Input: part model. Units: mm. Frame: model coordinates. A direction names the side the tool comes from. Coordinates: 2 decimals unless noted, no trailing zeros. Order: outer loops, then holes, each group sorted by start corner. A loop starts at its lowest first (then second) coordinate and runs counter-clockwise, first axis right, second up. Notation, with made-up numbers: (11, 48) -> (33, 48) arc R33 ccw to (33, 79) -> close; hole circle Ø1 at (28.25, 21). An arc over 180 degrees is marked (long way). Use one line per item in the form item = value. Start each with the question number.
1) Draft query along X for faces 1 (the flat face through (-133, 2, -17.245)), 2 (the flat face through (-2, 2, 4.205)), 3 (the flat face through (-46.62, 1.57, 10.22)). Return one class per face: pulls with the +X half, pulls with the -X half, needs draft (parallel to the pull), parting line crosses it, or undercut.
2) Access query for faces 4 (the flat face through (-122.093, 2, -2)), 5 (the flat face through (-79, 0, -2)). Directions: +Z, -Z, +X, -X, +Y, -Y. A direction counts if a zero-diameter tool reaches every point of the face in a straight line with its end or side. Return the directions, or none.
3) Section query B-B on z = -7. Output: boundary loops of the cut face in (x, y) (3 decimals).
4) Section query D-D on x = -36.5. Output: boundary loops of the cut face in (y, z) (3 decimals).
5) Section query A-A on x = -141. Output: boundary loops of the cut face in (y, z) (3 decimals).
6) Pin query (flat end, axial travel): pin 1 (7 mm diameter, centred on x = -168.39, z = -7.24, fed in from -Y); pin 2 (1 mm diameter, centred on y = 1.5, z = -4.5, fed in from +X); pin 3 (1.6 mm diameter, centred on y = 1, z = 2, fed in from -X); pin 4 (1 mm diameter, centred on x = -7, y = 2.5, fed in from -Z). Return the tip coordinate at first contact, or that it passes through.
7) Ray query, line 1 along Z through (x, y) = (-125.5, 2.35); line 2 along Z through (x, y) = (-117, 0.7); line 3 along X through (y, z) = (3.05, -9). Return the intervals inside material, ascending.
8) Section query C-C on y = 1.1. Count the separate pieces of the cut face and the enclosed holes in it, then the cut area to 3 significant figures.
from build123d import *

# Parameters (mm, degrees)
SKETCH1_R           = 2.25
SKETCH1_R_2         = 1
SKETCH1_W           = 40.6
SKETCH1_H           = 20.8
SKETCH1_W_2         = 23
SKETCH1_H_2         = 12.9
BOSS_EXTRUDE1_DEPTH = 3.175


with BuildPart() as part:
    # Sketch1 → Boss-Extrude1 (new body)
    with BuildSketch(Plane(origin=(0, 0, 0), x_dir=(1, 0, 0), z_dir=(0, 1, 0))):
        with BuildLine():
            Line((-162.38735588, 17.244652891), (-102.38735588, 17.244652891))
            Line((-102.38735588, 17.244652891), (7.61264412, 12.244652891))
            ThreePointArc((7.61264412, 12.244652891), (17.61264412, 2.244652891), (7.61264412, -7.755347109))
            Line((7.61264412, -7.755347109), (-102.38735588, -12.755347109))
            Line((-102.38735588, -12.755347109), (-162.38735588, -12.755347109))
            ThreePointArc((-162.38735588, -12.755347109), (-177.38735588, 2.244652891), (-162.38735588, 17.244652891))
        make_face()
        with Locations(Location((-168.38735588, 7.244652891, 0), (0, 0, 270))):
            Circle(SKETCH1_R, mode=Mode.SUBTRACT)
        with Locations(Location((-168.38735588, -2.755347109, 0), (0, 0, 270))):
            Circle(SKETCH1_R, mode=Mode.SUBTRACT)
        with Locations(Location((-118.78735588, 7.244652891, 0), (0, 0, 270))):
            Circle(SKETCH1_R, mode=Mode.SUBTRACT)
        with Locations(Location((-118.78735588, -2.755347109, 0), (0, 0, 270))):
            Circle(SKETCH1_R, mode=Mode.SUBTRACT)
        with Locations(Location((-15.58735588, 2.244652891, 0), (0, 0, 270))):
            Circle(SKETCH1_R_2, mode=Mode.SUBTRACT)
        with Locations(Location((11.81264412, 2.244652891, 0), (0, 0, 270))):
            Circle(SKETCH1_R_2, mode=Mode.SUBTRACT)
        with Locations(Location((-42.38735588, 2.244652891, 0), (0, 0, 270))):
            Circle(SKETCH1_R, mode=Mode.SUBTRACT)
        with Locations((-142.392621679, 2.244652891)):
            Rectangle(SKETCH1_W, SKETCH1_H, mode=Mode.SUBTRACT)
        with Locations((-1.88735588, 2.244652891)):
            Rectangle(SKETCH1_W_2, SKETCH1_H_2, mode=Mode.SUBTRACT)
    extrude(amount=BOSS_EXTRUDE1_DEPTH)


solid = part.part
Answers below:
q1.face_1 = needs draft
q1.face_2 = undercut
q1.face_3 = pulls with the +X half
q2.face_4 = +Y, -Y
q2.face_5 = +Z, -Z, +X, -X, -Y
q3.outline = (-176.614, 0) -> (-170.624, 0) -> (-170.624, 3.175) -> (-176.614, 3.175) -> close; (-166.151, 0) -> (-162.693, 0) -> (-162.693, 3.175) -> (-166.151, 3.175) -> close; (-122.093, 0) -> (-121.024, 0) -> (-121.024, 3.175) -> (-122.093, 3.175) -> close; (-116.551, 0) -> (-13.387, 0) -> (-13.387, 3.175) -> (-116.551, 3.175) -> close; (9.613, 0) -> (16.41, 0) -> (16.41, 3.175) -> (9.613, 3.175) -> close
q4.outline = (0, -14.25) -> (3.175, -14.25) -> (3.175, 9.76) -> (0, 9.76) -> close
q5.outline = (0, -17.245) -> (3.175, -17.245) -> (3.175, -12.645) -> (0, -12.645) -> close; (0, 8.155) -> (3.175, 8.155) -> (3.175, 12.755) -> (0, 12.755) -> close
q6.pin_1 = 0
q6.pin_2 = 17.46
q6.pin_3 = -176.99
q6.pin_4 = -12.93
q7.line_1 = -17.24 to -12.64, 8.16 to 12.76
q7.line_2 = -17.24 to -8.61, -5.88 to 1.39, 4.12 to 12.76
q7.line_3 = -175.78 to -169.79, -166.98 to -162.69, -122.09 to -120.19, -117.38 to 14.99
q8.separate_pieces = 1
q8.enclosed_holes = 9
q8.area = 3,830 mm^2
